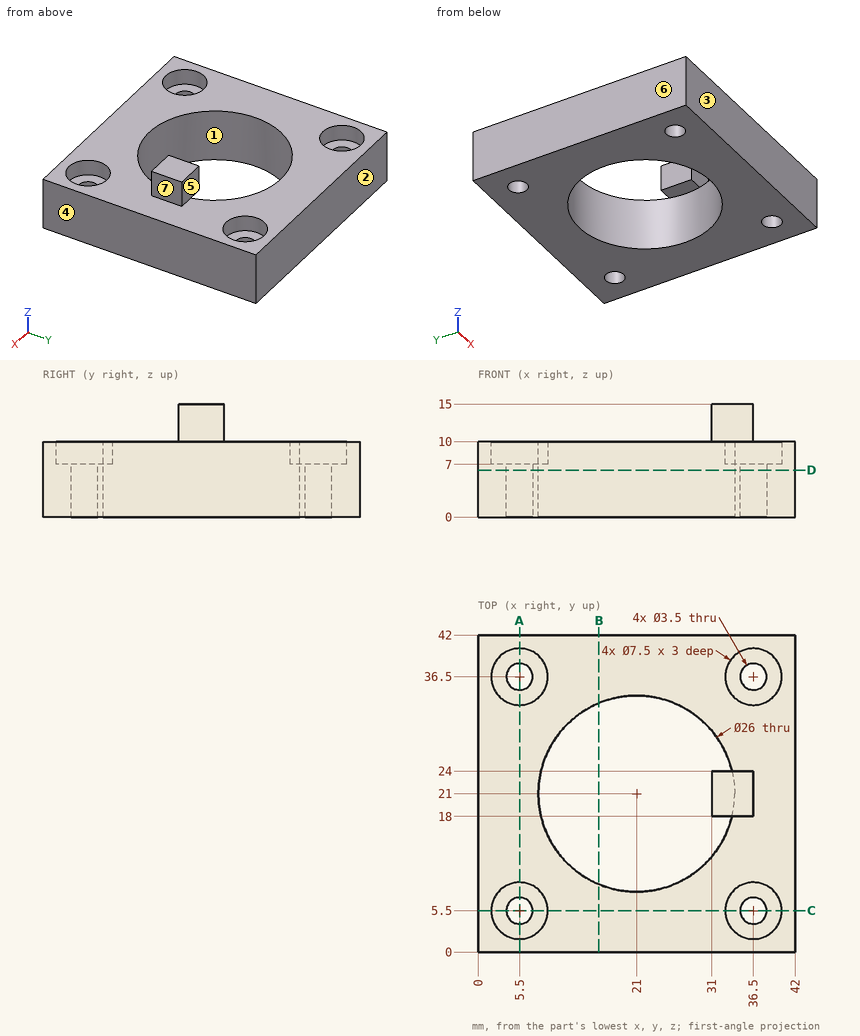
Drawing for the job (mm, zero at the part's lowest x, y, z). A direction names the side the tool comes from. Coordinates: 2 decimals unless noted, no trailing zeros. Write each loop counter-clockwise with the first axis right and the second up, starting at its lowest first coordinate (ties: lowest second). Pieces come first, ordered by that corner, then holes. Notation, with made-up numbers: (-4, 52) - (26, 52) arc R35 cw to (26, 91) - close; hole circle Ø6 at (-20.5, 8.25). An arc over 180 degrees is marked (long way). Write each question's results on one line, items separated by ' | '. Start each with the question number.
1) Mould opens along Y. For the marked faces 1, 2, 3 and 4 say: pulls with the +Y half, pulls with the -Y half, needs draft (parallel to the pull), parting line crosses it, or undercut.
2) Cut at B-B (x = 16). Write the cut outline in (y, z).
3) Flat gauge pins, fed straight in: P1, Ø10, axis at x = 10.5, y = 11, coming from the -Z side; P2, Ø1.5, axis at x = 34, z = 12, coming from the +Y side; P3, Ø4.5, axis at x = 36.5, y = 36.5, coming from the +Z side; P4, Ø2.5, axis at x = 33.5, z = 12.5, coming from the -Y side. Where does each tip first touch, or does it go through?
4) Cut at D-D (z = 6.25). Write the cut outline in (x, y), then the cut area to 3 significant figures.
5) Cut at A-A (x = 5.5). Write the cut outline in (y, z).
6) 3-axis set-ups, long thin cutter, end or side, ignore diameter. For the marked faces 5, 6 and 7: which of +Z, -Z, +X, -X, +Y, -Y reach the whole face in a straight line?
7) Probe line 1 along Y through (x, z) = (36.5, 2.5); line 2 along Y through (x, z) = (5.5, 8.75); line 3 along X through (y, z) = (4, 3). List the from-to ranges inside material, lowest first. Write a range as from..to.
Returned:
1) face 1: undercut | face 2: pulls with the +Y half | face 3: pulls with the -Y half | face 4: needs draft
2) outline: (0, 0) - (9, 0) - (9, 10) - (0, 10) - close; (33, 0) - (42, 0) - (42, 10) - (33, 10) - close
3) P1: z = 0 | P2: y = 24 | P3: z = 7 | P4: y = 18
4) outline: (0, 0) - (42, 0) - (42, 42) - (0, 42) - close; hole circle Ø3.5 at (5.5, 5.5); hole circle Ø3.5 at (5.5, 36.5); hole circle Ø26 at (21, 21); hole circle Ø3.5 at (36.5, 5.5); hole circle Ø3.5 at (36.5, 36.5) | area: 1,190 mm^2
5) outline: (0, 0) - (3.75, 0) - (3.75, 7) - (1.75, 7) - (1.75, 10) - (0, 10) - close; (7.25, 0) - (34.75, 0) - (34.75, 7) - (32.75, 7) - (32.75, 10) - (9.25, 10) - (9.25, 7) - (7.25, 7) - close; (38.25, 0) - (42, 0) - (42, 10) - (40.25, 10) - (40.25, 7) - (38.25, 7) - close
6) face 5: +Z, +X, -X, +Y | face 6: +Z, -Z, -X, +Y, -Y | face 7: +Z, +X, +Y, -Y
7) line 1: 0..3.75, 7.25..34.75, 38.25..42 | line 2: 0..1.75, 9.25..32.75, 40.25..42 | line 3: 0..4.6, 6.4..35.6, 37.4..42
